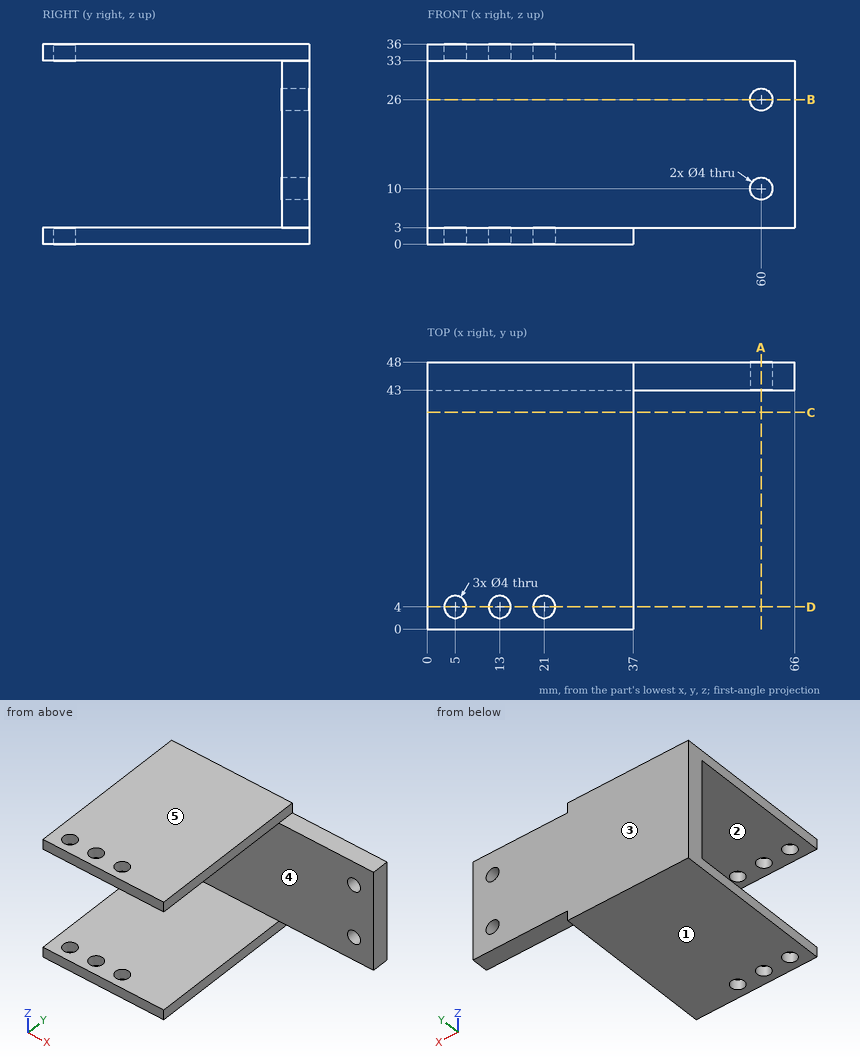
Design review of the part shown in the three views and the two pictorial views. Dimensions are in mm from the part's minimum x, y and z. A direction names the side the tool comes from. Coordinates: 2 decimals unless noted, no trailing zeros. Order: outer loops, then holes, each group sorted by start corner. A loop starts at its lowest first (then second) coordinate and runs counter-clockwise, first axis right, second up.
Item 1: For the marked faces 4 and 5, list the 3-axis set-ups (+Z, -Z, +X, -X, +Y, -Y) from which the entire face can be reached by the end or side of a thin tool; tool diameter is ignored.
Item 2: For pin 1 Ø1.5 at (x, y) = (49.5, 45.5) entering from +Z; pin 2 Ø10 at (y, z) = (18.5, 29.5) entering from +X; pin 3 Ø9 at (x, z) = (36.5, 19.5) entering from -Y, all flat-tipped, find the tip position at first contact; note any pin that passes through.
Item 3: For line 1 (Y direction, x = 13, z = 1); line 2 (X direction, y = 44.5, z = 10); line 3 (Z direction, x = 21, y = 7.5), list the stretches that pass through material, from the lowest coordinate up.
Item 4: The part is to be moulded in two halves that separate along Z. For the marked faces 1, 2 and 3, say which applies: pulls with the +Z half, pulls with the -Z half, needs draft (parallel to the pull), parting line crosses it, or undercut.
Item 5: Take a section at B-B, the plane z = 26. Write out the cut boundary in (x, y).
Item 6: Take a section at D-D, the plane y = 4. Count the separate pieces of the cut face and the enclosed holes in it, then the cut area to 3 significant figures.
Item 7: Take a section at A-A, the plane x = 60. Write out the cut boundary in (y, z).
Item 8: Take a section at C-C, the plane y = 39. Write out the cut boundary in (x, z).
The answers:
1. face 4: +X, -X, -Y
1. face 5: +Z, +X, -X, +Y, -Y
2. pin 1: stops at z = 33
2. pin 2: stops at x = 37
2. pin 3: stops at y = 43
3. line 1: y = 0 to 2, 6 to 48
3. line 2: x = 0 to 58, 62 to 66
3. line 3: z = 0 to 3, 33 to 36
4. face 1: pulls with the -Z half
4. face 2: undercut
4. face 3: needs draft
5. outline: (0, 43) - (58, 43) - (58, 48) - (0, 48) - close; (62, 43) - (66, 43) - (66, 48) - (62, 48) - close
6. separate pieces: 8
6. enclosed holes: 0
6. area: 150 mm2
7. outline: (43, 3) - (48, 3) - (48, 8) - (43, 8) - close; (43, 12) - (48, 12) - (48, 24) - (43, 24) - close; (43, 28) - (48, 28) - (48, 33) - (43, 33) - close
8. outline: (0, 0) - (37, 0) - (37, 3) - (0, 3) - close; (0, 33) - (37, 33) - (37, 36) - (0, 36) - close
